Could you check a few things on this drawing? It's one solid part, dimensions in mm from its lowest x, y, z. Give positions to 0.01 mm unless a question says otherwise; leave off trailing zeros. Order: outer loops, then holes, each group sorted by start corner. A loop starts at its lowest first (then second) coordinate and runs counter-clockwise, first axis right, second up. Notation, with made-up numbers: M -33,19.5 L -15,19.5 A12 ccw -15,26.5 Z; hole C -39,-4.75 d6. An arc over 180 degrees is marked long. Return JSON: item names as keys, results as strings. Group by question number.
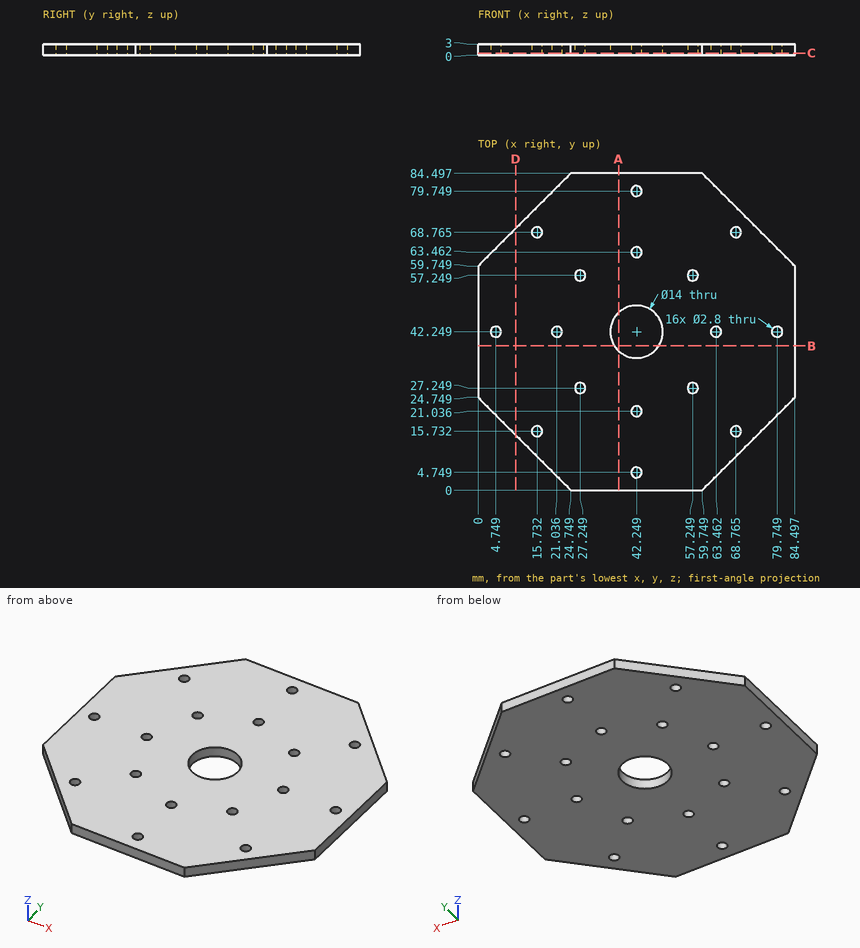
1. Imagine slicing it at D-D, the plane x = 10. Please give me the cut outline in (y, z), plus the area to 3 significant figures.
2. Imagine slicing it at A-A, the plane x = 37.5. Please give me the cut outline in (y, z) (1 decimal).
3. Imagine slicing it at C-C, the plane z = 0.6. Count the separate pieces of the cut face and the enclosed holes in it, plus the area to 3 significant figures.
4. For pin 1 (2 mm diameter, centred on x = 42.25, y = 79.75, fed in from +Z); pin 2 (1.5 mm diameter, centred on y = 19, z = 2, fed in from -X), each with a flat end and sliding along its axis, tell me the tip position at first contact or that it passes through.
5. Imagine slicing it at B-B, the plane y = 38.5. Please give me the cut outline in (x, z), plus the area to 3 significant figures.
6. I need wall thicknesses on L1, parallel to Y at x = 57.5, z = 2.75 (1 decimal); L2, parallel to Y at x = 40, z = 2; L3, parallel to Y at x = 36, z = 1.55 (1 decimal). Which ranges of each line are inside material? Lowest first, please. Write a range as from..to.
Values:
{
 "1": {"outline": "M 14.75,0 L 69.75,0 L 69.75,3 L 14.75,3 Z", "area": "165 mm²"},
 "2": {"outline": "M 0,0 L 37.1,0 L 37.1,3 L 0,3 Z; M 47.4,0 L 84.5,0 L 84.5,3 L 47.4,3 Z"},
 "3": {"separate pieces": "1", "enclosed holes": "17", "area": "5,660 mm²"},
 "4": {"pin 1": "passes through", "pin 2": "stops at x = 5"},
 "5": {"outline": "M 0,0 L 36.34,0 L 36.34,3 L 0,3 Z; M 48.16,0 L 84.5,0 L 84.5,3 L 48.16,3 Z", "area": "218 mm²"},
 "6": {"L1": "y = 0..25.9, 28.6..55.9, 58.6..84.5", "L2": "y = 0..35.62, 48.88..84.5", "L3": "y = 0..39.1, 45.4..84.5"}
}
